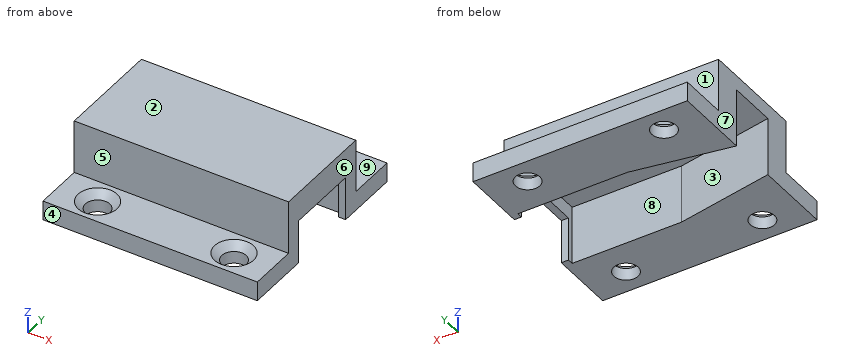
```python
from build123d import *

# Parameters (mm, degrees)
SKETCH001_W     = 44
SKETCH001_H     = 41.5
PAD_DEPTH       = 15
POCKET_DEPTH    = 12
SKETCH002_W     = 15
SKETCH002_H     = 9
POCKET001_DEPTH = 5
SKETCH003_W     = 44
SKETCH003_H     = 10
POCKET002_DEPTH = 11
SKETCH004_R     = 2.5
POCKET003_DEPTH = 5
CHAMFER_SIZE    = 1.5


with BuildPart() as part:
    # Sketch001 → Pad (new body)
    with BuildSketch(Plane.XY):
        Rectangle(SKETCH001_W, SKETCH001_H)
    extrude(amount=PAD_DEPTH)

    # Sketch (on Face5 of Pad) → Pocket (cut)
    with BuildSketch(Plane(origin=(0, 0, 0), x_dir=(1, 0, 0), z_dir=(0, 0, -1))):
        Polygon((20.53, 8.680906), (-1.95, 8.680906), (-22, 5.009672), (-22, -4.990328), (-1.949989, -8.661501), (20.53, -8.639094), align=None)
    extrude(amount=-POCKET_DEPTH, mode=Mode.SUBTRACT)

    # Sketch002 (on Face3 of Pocket) → Pocket001 (cut)
    with BuildSketch(Plane.YZ.offset(22)):
        with Locations((0, 4.5)):
            Rectangle(SKETCH002_W, SKETCH002_H)
    extrude(amount=-POCKET001_DEPTH, mode=Mode.SUBTRACT)

    # Sketch003 (on Face5 of Pocket001) → Pocket002 (cut)
    with BuildSketch(Plane.XY.offset(15)):
        with Locations((0, -15.75)):
            Rectangle(SKETCH003_W, SKETCH003_H)
        with Locations((0, 15.75)):
            Rectangle(SKETCH003_W, SKETCH003_H)
    extrude(amount=-POCKET002_DEPTH, mode=Mode.SUBTRACT)

    # Sketch004 (on Face14 of Pocket002) → Pocket003 (cut)
    with BuildSketch(Plane.XY.offset(4)):
        with Locations((-14, -15.75)):
            Circle(SKETCH004_R)
        with Locations((14, -15.75)):
            Circle(SKETCH004_R)
        with Locations((-14, 15.75)):
            Circle(SKETCH004_R)
        with Locations((14, 15.75)):
            Circle(SKETCH004_R)
    extrude(amount=-POCKET003_DEPTH, mode=Mode.SUBTRACT)

    # Chamfer
    chamfer_edges = [part.edges().sort_by_distance(p)[0] for p in [
        (11.5, -15.75, 4),
        (-16.5, -15.75, 4),
        (-16.5, 15.75, 4),
        (11.5, 15.75, 4),
    ]]
    chamfer(chamfer_edges, length=CHAMFER_SIZE)


solid = part.part
```
Design review of the part built by this model. Coordinates are the model's own, in mm. Face numbers are marked on the shaded views. A direction names the side the tool comes from. Give positions to 0.01 mm unless a question says otherwise; leave off trailing zeros. Loops run counter-clockwise (first coordinate to the right, second up) from the corner with the lowest first, then second, coordinate; pieces in that order, holes last. Notation, with made-up numbers: M 31,59.25 L 84,59.25 A25 ccw 84,93.25 Z; hole C 65,24.25 d5. An arc over 180 degrees is marked long. Return JSON: item names as keys, results as strings. Group by question number.
Item 1: We need section A-A (y = -15.75). Give the boundary of the cut face in (x, z).
Item 2: Mouldability with a two-part tool opening along X and no side actions: class the marked faces 6, 7, 8 and 9 as released by +X, released by -X, zero draft, split by the parting line, or undercut.
Item 3: For probe 1 along Y at (x, z) = (14, 1.65); probe 2 along Y at (x, z) = (2.5, 7.25); probe 3 along Y at (x, z) = (-14, 0.85), list the stretches that pass through material, from the lowest coordinate up.
Item 4: We need section B-B (x = 14). Give the boundary of the cut face in (y, z).
Item 5: We need section D-D (y = 3). Give the boundary of the cut face in (x, z), and give its area (3 significant figures).
Item 6: Tool access review of the marked faces 1, 2, 3, 4 and 5: name each direction out of +Z, -Z, +X, -X, +Y, -Y from which nothing blocks a thin tool from reaching the whole face with its end or side.
Item 7: Insertion check: pin 1 Ø5 at (x, y) = (-1.5, 17) entering from +Z; pin 2 Ø4 at (x, z) = (17, 10) entering from -Y; pin 3 Ø9 at (x, z) = (-4.5, 10.5) entering from +Y; pin 4 Ø1.5 at (x, y) = (-14, -14.5) entering from +Z. Each pin has a flat end and moves straight along its axis. Give the tip position at first contact, or say it passes through.
Item 8: We need section C-C (z = 11.5). Give the boundary of the cut face in (x, y), and give its area (3 significant figures).
Output:
{
 "1": {"outline": "M -22,0 L -16.5,0 L -16.5,2.5 L -18,4 L -22,4 Z; M -11.5,0 L 11.5,0 L 11.5,2.5 L 10,4 L -10,4 L -11.5,2.5 Z; M 16.5,0 L 22,0 L 22,4 L 18,4 L 16.5,2.5 Z"},
 "2": {"face 6": "released by +X", "face 7": "released by -X", "face 8": "undercut", "face 9": "zero draft"},
 "3": {"probe 1": "y = -20.75 to -18.25, -13.25 to -8.68, 8.65 to 13.25, 18.25 to 20.75", "probe 2": "y = -10.75 to -8.68, 8.66 to 10.75", "probe 3": "y = -20.75 to -18.25, -13.25 to -6.47, 6.46 to 13.25, 18.25 to 20.75"},
 "4": {"outline": "M -20.75,0 L -18.25,0 L -18.25,2.5 L -19.75,4 L -20.75,4 Z; M -13.25,0 L -8.68,0 L -8.68,12 L 8.65,12 L 8.65,0 L 13.25,0 L 13.25,2.5 L 11.75,4 L 10.75,4 L 10.75,15 L -10.75,15 L -10.75,4 L -11.75,4 L -13.25,2.5 Z; M 18.25,0 L 20.75,0 L 20.75,4 L 19.75,4 L 18.25,2.5 Z"},
 "5": {"outline": "M -22,12 L 20.53,12 L 20.53,9 L 22,9 L 22,15 L -22,15 Z", "area": "136 mm^2"},
 "6": {"face 1": "+Z, +X, -X, +Y", "face 2": "+Z, +X, -X, +Y, -Y", "face 3": "-Z", "face 4": "+Z, -Z, +X, -X, -Y", "face 5": "+Z, +X, -X, -Y"},
 "7": {"pin 1": "stops at z = 4", "pin 2": "stops at y = -10.75", "pin 3": "stops at y = 10.75", "pin 4": "passes through"},
 "8": {"outline": "M -22,-10.75 L 22,-10.75 L 22,10.75 L -22,10.75 L -22,4.99 L -1.95,8.66 L 20.53,8.64 L 20.53,-8.68 L -1.95,-8.68 L -22,-5.01 Z", "area": "282 mm^2"}
}
